from build123d import *

# Parameters (mm, degrees)
BOSS_EXTRUDE1_DEPTH = 60
SKETCH3_W           = 30
SKETCH3_H           = 20
BOSS_EXTRUDE2_DEPTH = 80
SKETCH4_W           = 40
SKETCH4_H           = 15
CUT_EXTRUDE1_DEPTH  = 141.678348685
BOSS_EXTRUDE3_DEPTH = 30
BOSS_EXTRUDE4_DEPTH = 30
SKETCH8_W           = 10
SKETCH8_H           = 35
CUT_EXTRUDE2_DEPTH  = 61
SKETCH9_W           = 10
SKETCH9_H           = 35
CUT_EXTRUDE3_DEPTH  = 61
SKETCH10_R          = 7
CUT_EXTRUDE4_DEPTH  = 61
SKETCH12_R          = 10
CUT_EXTRUDE5_DEPTH  = 12
SKETCH13_R          = 15
CUT_EXTRUDE6_DEPTH  = 12


with BuildPart() as part:
    # Sketch1 → Boss-Extrude1 (new body)
    with BuildSketch(Plane(origin=(0, 0, 0), x_dir=(1, 0, 0), z_dir=(0, 1, 0))):
        Polygon((-7.906128035, 42.313092402), (-17.906128035, 42.313092402), (-17.906128035, -37.686907598), (-7.906128035, -37.686907598), (-7.906128035, -22.686907598), (32.093871965, -22.686907598), (32.093871965, -37.686907598), (42.093871965, -37.686907598), (42.093871965, 42.313092402), (32.093871965, 42.313092402), (32.093871965, 27.313092402), (-7.906128035, 27.313092402), align=None)
    extrude(amount=-BOSS_EXTRUDE1_DEPTH)

    # Sketch3 → Boss-Extrude2 (add)
    with BuildSketch(Plane.XY.offset(37.686907598)):
        with Locations((-32.906128035, -50)):
            Rectangle(SKETCH3_W, SKETCH3_H)
        with Locations((57.093871965, -50)):
            Rectangle(SKETCH3_W, SKETCH3_H)
    extrude(amount=-BOSS_EXTRUDE2_DEPTH)

    # Sketch4 → Cut-Extrude1 (cut, through all)
    with BuildSketch(Plane.ZY.offset(47.906128035)):
        with Locations((-2.313092402, -52.5)):
            Rectangle(SKETCH4_W, SKETCH4_H)
    extrude(amount=-CUT_EXTRUDE1_DEPTH, mode=Mode.SUBTRACT)

    # Sketch5 → Boss-Extrude3 (add)
    with BuildSketch(Plane.ZY.offset(47.906128035)):
        Polygon((-42.313092402, -40), (-2.313092402, 0), (37.686907598, -40), align=None)
    extrude(amount=-BOSS_EXTRUDE3_DEPTH)

    # Sketch6 → Boss-Extrude4 (add)
    with BuildSketch(Plane(origin=(72.093871965, 0, 0), x_dir=(0, 0, -1), z_dir=(1, 0, 0))):
        Polygon((-37.686907598, -40), (2.313092402, 0), (42.313092402, -40), align=None)
    extrude(amount=-BOSS_EXTRUDE4_DEPTH)

    # Sketch8 → Cut-Extrude2 (cut, symmetric)
    with BuildSketch(Plane.XY.offset(-2.313092402)):
        with Locations((-32.906128035, -17.5)):
            Rectangle(SKETCH8_W, SKETCH8_H)
    extrude(amount=CUT_EXTRUDE2_DEPTH, both=True, mode=Mode.SUBTRACT)

    # Sketch9 → Cut-Extrude3 (cut, symmetric)
    with BuildSketch(Plane.XY.offset(-2.313092402)):
        with Locations((57.093871965, -17.5)):
            Rectangle(SKETCH9_W, SKETCH9_H)
    extrude(amount=CUT_EXTRUDE3_DEPTH, both=True, mode=Mode.SUBTRACT)

    # Sketch10 → Cut-Extrude4 (cut, symmetric)
    with BuildSketch(Plane.XY.offset(22.686907598)):
        with Locations((12.093871965, -30)):
            Circle(SKETCH10_R)
    extrude(amount=CUT_EXTRUDE4_DEPTH, both=True, mode=Mode.SUBTRACT)

    # Sketch12 → Cut-Extrude5 (cut)
    with BuildSketch(Plane(origin=(0, -10, 0), x_dir=(1, 0, 0), z_dir=(0, 1, 0))):
        with Locations(Location((12.093871965, 2.313092402, 0), (0, 0, 270))):
            Circle(SKETCH12_R)
    extrude(amount=-CUT_EXTRUDE5_DEPTH, mode=Mode.SUBTRACT)

    # Sketch13 → Cut-Extrude6 (cut)
    with BuildSketch(Plane(origin=(0, 0, 0), x_dir=(1, 0, 0), z_dir=(0, 1, 0))):
        with Locations(Location((12.093871965, 2.313092402, 0), (0, 0, 270))):
            Circle(SKETCH13_R)
    extrude(amount=-CUT_EXTRUDE6_DEPTH, mode=Mode.SUBTRACT)


solid = part.part
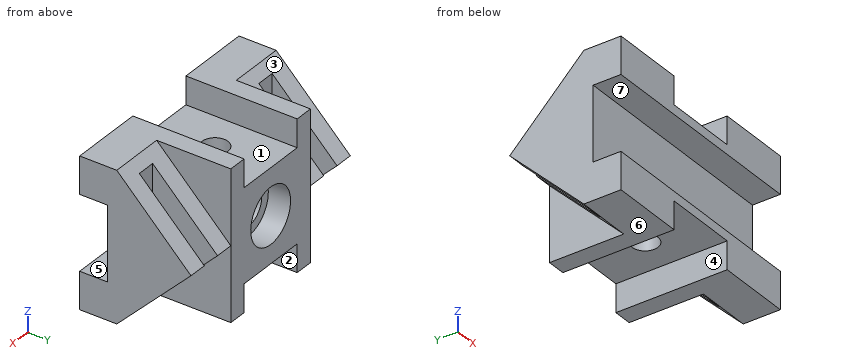
Could you check a few things on this model? Use its own coordinates, in mm. Face numbers are marked on the shaded views. A direction names the side the tool comes from. Round coordinates to 2 decimals unless told otherwise and drop trailing zeros. Order: outer loops, then holes, each group sorted by start corner. A loop starts at its lowest first (then second) coordinate and runs counter-clockwise, first axis right, second up.
Q1. Imagine slicing it at C-C, the plane z = 24. List the corners of the cut face in (x, y) for me, then the cut area to 3 significant figures.
Geometry says:
outline: (-47.91, -60) - (-7.91, -60) - (-7.91, 0) - (-17.91, 0) - (-17.91, -26.31) - (-27.91, -26.31) - (-27.91, -35) - (-37.91, -35) - (-37.91, -26.31) - (-47.91, -26.31) - close; (32.09, -60) - (72.09, -60) - (72.09, -26.31) - (62.09, -26.31) - (62.09, -35) - (52.09, -35) - (52.09, -26.31) - (42.09, -26.31) - (42.09, 0) - (32.09, 0) - close
area: 3,050 mm2
Q2. I'm going to push flat-ended pins straight in: P1, Ø7.5, axis at y = -16.5, z = 32, coming from the -X side; P2, Ø2, axis at x = 30, z = -28, coming from the -Y side; P3, Ø3, axis at x = -4, z = -15.5, coming from the -Y side; P4, Ø4, axis at x = -1, y = -28, coming from the +Z side. Where does each tip first touch, or does it pass through?
Geometry says:
P1: stops at x = -17.91
P2: stops at y = -60
P3: stops at y = -45
P4: stops at z = 22.69
Q3. Imagine slicing it at B-B, the plane x = 48. List the corners of the cut face in (y, z) for me.
Geometry says:
outline: (-60, -42.31) - (-40, -42.31) - (0, -2.31) - (-40, 37.69) - (-60, 37.69) - (-60, 17.69) - (-45, 17.69) - (-45, -22.31) - (-60, -22.31) - close
Q4. Please list where these lines run through material, in increasing order: probe 1 along X at (y, z) = (-22.5, 11); probe 2 along Y at (x, z) = (12, -15); probe 3 along X at (y, z) = (-8.5, 34.5).
Geometry says:
probe 1: x = -47.91 to -37.91, -27.91 to 52.09, 62.09 to 72.09
probe 2: y = -45 to -37, -23 to -12
probe 3: x = -17.91 to -7.91, 32.09 to 42.09
Q5. Which directions (+Z, -Z, +X, -X, +Y, -Y) give clear straight access to the entire face, cutting with the end or side of a thin tool? Please do the marked faces 1, 2 and 3.
Geometry says:
face 1: +Z, +Y, -Y
face 2: -Z, +Y, -Y
face 3: +Z, -X, +Y
Q6. Imagine slicing it at A-A, the plane y = -3.5. State how many separate pieces and enclosed holes the cut face has, then the cut area to 3 significant figures.
Geometry says:
separate pieces: 3
enclosed holes: 1
area: 3,170 mm2
Q7. Thinking about a two-plate mould opening in Z: for the marked faces 4, 5, 6 and 7, which applies, released by +Z, released by -Z, zero draft, split by the parting line, or undercut?
Geometry says:
face 4: zero draft
face 5: undercut
face 6: released by -Z
face 7: undercut
